The model under review builds one solid part; all positions refer to its coordinate system, in mm. A direction names the side the tool comes from. Coordinates: 2 decimals unless noted, no trailing zeros. Order: outer loops, then holes, each group sorted by start corner. A loop starts at its lowest first (then second) coordinate and runs counter-clockwise, first axis right, second up.
from build123d import *

# Parameters (mm, degrees)
F1_DEPTH  = 2
F3_DEPTH  = 2.001
F4_W      = 3
F4_H      = 69.7761774063
F5_DEPTH  = 3
F7_D      = 6.6
F9_DEPTH  = 25
F10_W     = 25
F10_H     = 2.5
F11_DEPTH = 2


with BuildPart() as f1:
    # F0 (on Front) → F1 (new body)
    with BuildSketch(Plane.XZ):
        Polygon((-307.3464844827, 210.4111198679), (-307.3464844827, -195.9888801321), (200.6535155173, -195.9888801321), (200.6535155173, 210.4111198679), (149.8535155173, 312.0111198679), (-256.5464844827, 312.0111198679), align=None)
    extrude(amount=F1_DEPTH)

    # F2 (on face) → F3 (cut, through all)
    with BuildSketch(Plane.XZ.offset(2)):
        with BuildLine():
            Line((99.0535155173, 210.4111198679), (-205.7464844827, 210.4111198679))
            ThreePointArc((-205.7464844827, 210.4111198679), (-241.667508967, 195.5321443521), (-256.5464844827, 159.6111198679))
            Line((-256.5464844827, 159.6111198679), (-256.5464844827, -94.3888801321))
            ThreePointArc((-256.5464844827, -94.3888801321), (-241.667508967, -130.3099046164), (-205.7464844827, -145.1888801321))
            Line((-205.7464844827, -145.1888801321), (99.0535155173, -145.1888801321))
            ThreePointArc((99.0535155173, -145.1888801321), (134.9745400016, -130.3099046164), (149.8535155173, -94.3888801321))
            Line((149.8535155173, -94.3888801321), (149.8535155173, 159.6111198679))
            ThreePointArc((149.8535155173, 159.6111198679), (134.9745400016, 195.5321443521), (99.0535155173, 210.4111198679))
        make_face()
    extrude(amount=-F3_DEPTH, mode=Mode.SUBTRACT)

    # F4 (on face) → F5 (join)
    with BuildSketch(Plane.XZ.offset(2)):
        with Locations((-21.4731446389, 260.3619992733)):
            Rectangle(F4_W, F4_H)
    extrude(amount=-F5_DEPTH)

    # F7 (through all)
    with Locations(Plane.XZ.offset(2)):
        with Locations((-294.8464844827, 185.0111198679), (-294.8464844827, 7.2111198679), (-294.8464844827, -170.5888801321), (188.1535155173, -170.5888801321), (188.1535155173, 7.2111198679), (188.1535155173, 185.0111198679)):
            Hole(F7_D / 2)

    # F8 (on face) → F9 (cut)
    with BuildSketch(Plane.XZ.offset(2)):
        with BuildLine():
            Line((-284.9858047077, 199.2307799804), (-307.3464844827, 210.4111198679))
            Line((-307.3464844827, 210.4111198679), (-307.3464844827, -195.9888801321))
            Line((-307.3464844827, -195.9888801321), (200.6535155173, -195.9888801321))
            Line((200.6535155173, -195.9888801321), (200.6535155173, 210.4111198679))
            Line((200.6535155173, 210.4111198679), (178.2928357423, 199.2307799804))
            Line((178.2928357423, 199.2307799804), (135.7846318098, 284.2471878454))
            ThreePointArc((135.7846318098, 284.2471878454), (133.9411514154, 286.2643739096), (131.3124958548, 287.0111198679))
            Line((131.3124958548, 287.0111198679), (-238.0054648202, 287.0111198679))
            ThreePointArc((-238.0054648202, 287.0111198679), (-240.6341203808, 286.2643739096), (-242.4776007752, 284.2471878454))
            Line((-242.4776007752, 284.2471878454), (-284.9858047077, 199.2307799804))
        make_face()
    extrude(amount=-F9_DEPTH, mode=Mode.SUBTRACT)

    # F10 (on face) → F11 (join)
    with BuildSketch(Plane.XZ.offset(2)):
        with Locations((-194.0464844827, 313.2611198679)):
            Rectangle(F10_W, F10_H)
        with Locations((87.3535155173, 313.2611198679)):
            Rectangle(F10_W, F10_H)
        Polygon((-284.9858047077, 255.1324794179), (-273.8054648202, 277.4931591929), (-276.0415327977, 278.6111931816), (-287.2218726852, 256.2505134066), align=None)
        Polygon((169.3485638323, 278.6111931816), (167.1124958548, 277.4931591929), (178.2928357423, 255.1324794179), (180.5289037198, 256.2505134066), align=None)
    extrude(amount=-F11_DEPTH)


solid = f1.part
(1) Consider section C-C (x = 110). Give the boundary of the cut face in (y, z), then the cut area to 3 significant figures.
(2) Insertion check: pin 1 Ø1.5 at (y, z) = (-0.5, 277) entering from +X; pin 2 Ø1.6 at (x, y) = (122.5, -1) entering from +Z; pin 3 Ø0.6 at (y, z) = (-1, 314) entering from +X. Each pin has a flat end and moves straight along its axis. Give the tip position at first contact, or say it passes through.
(3) Tool access review of faces 1 (the face through (-263.434, -1.014, 242.334)), 2 (the face through (-281.55, -1.01, 267.59)): name each direction out of +Z, -Z, +X, -X, +Y, -Y from which nothing blocks a thin tool from reaching the whole face with its end or side.
(4) Consider section D-D (z = 261). Give the boundary of the cut face in (x, y), then the cut area to 3 significant figures.
(5) Consider section B-B (y = -0.7). Give the boundary of the cut face in (x, z).
(6) Consider section A-A (z = 229.5). Give the boundary of the cut face in (x, y).
(7) Wall thickness on line 1 (Y direction, x = -254, z = 299.5); line 2 (Z direction, x = -21, y = -0.85); line 3 (X direction, y = -1, z = 225.5): over which ranges is each line inside the solid? List them lowest first.
Findings:
1. outline: (-2, 287.01) - (0, 287.01) - (0, 312.01) - (-2, 312.01) - close
1. area: 50.0 mm2
2. pin 1: stops at x = 170.53
2. pin 2: stops at z = 312.01
2. pin 3: stops at x = 99.85
3. face 1: -Z, +Y, -Y
3. face 2: +Z, -X, +Y, -Y
4. outline: (-284.85, -2) - (-254.1, -2) - (-254.1, 0) - (-284.85, 0) - close; (147.41, -2) - (178.15, -2) - (178.15, 0) - (147.41, 0) - close
4. area: 123 mm2
5. outline: (-307.35, 210.41) - (-284.99, 199.23) - (-242.48, 284.25) arc R5 cw to (-238.01, 287.01) - (131.31, 287.01) arc R5 cw to (135.78, 284.25) - (178.29, 199.23) - (200.65, 210.41) - (178.29, 255.13) - (180.53, 256.25) - (169.35, 278.61) - (167.11, 277.49) - (149.85, 312.01) - (99.85, 312.01) - (99.85, 314.51) - (74.85, 314.51) - (74.85, 312.01) - (-181.55, 312.01) - (-181.55, 314.51) - (-206.55, 314.51) - (-206.55, 312.01) - (-256.55, 312.01) - (-273.81, 277.49) - (-276.04, 278.61) - (-287.22, 256.25) - (-284.99, 255.13) - close
6. outline: (-297.8, -2) - (-269.85, -2) - (-269.85, 0) - (-297.8, 0) - close; (163.16, -2) - (191.11, -2) - (191.11, 0) - (163.16, 0) - close
7. line 1: y = -2 to 0
7. line 2: z = 287.01 to 312.01
7. line 3: x = -299.8 to -271.85, 165.16 to 193.11
